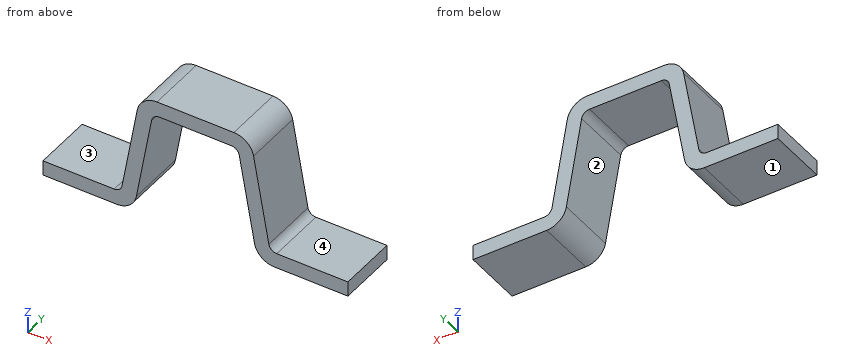
from build123d import *

# Parameters (mm, degrees)
F1_DEPTH = 38.1
F2_R     = 5.08
F3_R     = 12.7


with BuildPart() as f1:
    # F0 (on Front) → F1 (new body)
    with BuildSketch(Plane.XZ):
        Polygon((39.395954, -39.6875), (96.8375, -39.6875), (96.8375, -30.1625), (47.388378, -30.1625), (35.071938, 39.6875), (-35.071938, 39.6875), (-47.388378, -30.1625), (-96.8375, -30.1625), (-96.8375, -39.6875), (-39.395954, -39.6875), (-37.71644, -30.1625), (-27.079514, 30.1625), (27.079514, 30.1625), (37.71644, -30.1625), align=None)
    extrude(amount=F1_DEPTH)

    # F2
    f2_edges = [f1.edges().sort_by_distance(p)[0] for p in [
        (-27.079514, -19.05, 30.1625),
        (27.079514, -19.05, 30.1625),
        (47.388378, -19.05, -30.1625),
        (-47.388378, -19.05, -30.1625),
    ]]
    fillet(f2_edges, radius=F2_R)

    # F3
    f3_edges = [f1.edges().sort_by_distance(p)[0] for p in [
        (-39.395954, -19.05, -39.6875),
        (39.395954, -19.05, -39.6875),
        (35.071938, -19.05, 39.6875),
        (-35.071938, -19.05, 39.6875),
    ]]
    fillet(f3_edges, radius=F3_R)


solid = f1.part
Can you work these out from the model? Positions are in its coordinate system, mm. Face numbers are marked on the shaded views. A direction names the side the tool comes from. Give positions to 0.01 mm unless a question says otherwise; leave off trailing zeros. Write each loop counter-clockwise with the first axis right and the second up, starting at its lowest first coordinate (ties: lowest second). Pieces come first, ordered by that corner, then holes. Notation, with made-up numbers: (9, 75) -> (29, 75) arc R21 cw to (29, 81) -> close; hole circle Ø3 at (40.5, 20.5). An arc over 180 degrees is marked (long way). Answer as a JSON object with one key per item and string values. Group by question number.
Item 1: Please list where these lines run through material, in increasing order: line 1 (Z direction, x = -52.5, y = -23.5); line 2 (Z direction, x = -15, y = -8); line 3 (X direction, y = -21, z = -8). Write a range as [from, to].
Item 2: Suppose I cut it at A-A (z = -20.5). Please give me the cut outline in (x, y).
Item 3: Suppose I cut it at C-C (z = 33.5). Please give me the cut outline in (x, y).
Item 4: Suppose I cut it at B-B (x = -16). Please give me the cut outline in (y, z), plus the area to 3 significant figures.
Item 5: I'm going to push flat-ended pins straight in: P1, Ø12, axis at y = -8, z = 1.5, coming from the -X side; P2, Ø6, axis at y = -32, z = 23.5, coming from the -X side; P3, Ø3, axis at x = 65.5, y = -18, coming from the +Z side. Where does each tip first touch, or does it pass through?
Item 6: For the marked faces 1, 2, 3 and 4, which set-ups out of +Z, -Z, +X, -X, +Y, -Y let a thin tool reach every point of the face, with its end or its side?
Findings:
{
 "1": {"line 1": "z = [-39.69, -30.16]", "line 2": "z = [30.16, 39.69]", "line 3": "x = [-43.48, -33.81], [33.81, 43.48]"},
 "2": {"outline": "(-45.68, -38.1) -> (-36.01, -38.1) -> (-36.01, 0) -> (-45.68, 0) -> close; (36.01, -38.1) -> (45.68, -38.1) -> (45.68, 0) -> (36.01, 0) -> close"},
 "3": {"outline": "(-35.32, -38.1) -> (35.32, -38.1) -> (35.32, 0) -> (-35.32, 0) -> close"},
 "4": {"outline": "(-38.1, 30.16) -> (0, 30.16) -> (0, 39.69) -> (-38.1, 39.69) -> close", "area": "363 mm²"},
 "5": {"P1": "stops at x = -42.86", "P2": "stops at x = -38.46", "P3": "stops at z = -30.16"},
 "6": {"face 1": "-Z, +X, -X, +Y, -Y", "face 2": "-Z, +Y, -Y", "face 3": "+Z, -X, +Y, -Y", "face 4": "+Z, +X, +Y, -Y"}
}
